The model under review builds one solid part; all positions refer to its coordinate system, in mm. A direction names the side the tool comes from. Coordinates: 2 decimals unless noted, no trailing zeros. Write each loop counter-clockwise with the first axis right and the second up, starting at its lowest first coordinate (ties: lowest second). Pieces come first, ordered by that corner, then holes. Notation, with made-up numbers: M -1,80.25 L 15,80.25 A22 cw 15,116.25 Z; hole C -12,73 d10. An arc over 180 degrees is marked long. Answer as CSV lines item,"result". Start each with the question number.
from build123d import *

# Parameters (mm, degrees)
BOX002_W          = 25
BOX002_H          = 10
BOX002_DEPTH      = 25.45
BOX010_W          = 25
BOX010_H          = 1
BOX010_DEPTH      = 25.45
BOX_W             = 25
BOX_H             = 20
BOX_DEPTH         = 12
CYLINDER_R        = 51.5
CYLINDER_DEPTH    = 16
CYLINDER001_R     = 53.5
CYLINDER001_DEPTH = 16


with BuildPart() as cube002:
    # Box002 → Box002 (new body)
    with BuildSketch(Plane(origin=(40, -5, 2.55), x_dir=(1, 0, 0), z_dir=(0, 0, 1))):
        with Locations((12.5, 5)):
            Rectangle(BOX002_W, BOX002_H)
    extrude(amount=BOX002_DEPTH)


with BuildPart() as cube010:
    # Box010 → Box010 (new body)
    with BuildSketch(Plane(origin=(45, -0.5, -3.45), x_dir=(1, 0, 0), z_dir=(0, 0, 1))):
        with Locations((12.5, 0.5)):
            Rectangle(BOX010_W, BOX010_H)
    extrude(amount=BOX010_DEPTH)


with BuildPart() as obj1:
    # Box → Box (new body)
    with BuildSketch(Plane(origin=(40, -10, 2), x_dir=(1, 0, 0), z_dir=(0, 0, 1))):
        with Locations((12.5, 10)):
            Rectangle(BOX_W, BOX_H)
    extrude(amount=BOX_DEPTH)

    # Fusion: union Cube002, Cube010
    add(cube002.part)
    add(cube010.part)


with BuildPart() as cylinder_chico:
    # Cylinder → Cylinder (new body)
    with BuildSketch(Plane.XY):
        Circle(CYLINDER_R)
    extrude(amount=CYLINDER_DEPTH)


with BuildPart() as cut015021:
    # Cylinder001 → Cylinder001 (new body)
    with BuildSketch(Plane.XY):
        Circle(CYLINDER001_R)
    extrude(amount=CYLINDER001_DEPTH)

    # Cut: cut Cylinder_chico
    add(cylinder_chico.part, mode=Mode.SUBTRACT)

    # Cut015021: cut obj1
    add(obj1.part, mode=Mode.SUBTRACT)


solid = cut015021.part
1) To check wall thickness, follow line 1 (Y direction, x = 0, z = 10.25); line 2 (X direction, y = -25.5, z = 9); line 3 (X direction, y = 0, z = 10.75). State the ranges of each line that lie inside material, in increasing order. Write a range as [from, to].
2) Clearance check with flat-ended pins moving along their axes: pin 1 Ø0.9 at (x, y) = (52, 3.5) entering from +Z; pin 2 Ø2 at (x, y) = (51.5, -8) entering from -Z; pin 3 Ø3 at (y, z) = (28.5, 5.5) entering from -X; pin 4 Ø2 at (y, z) = (-3.5, 11.5) entering from -X. State where each tip first meets the part, or that it passes through.
3) Mouldability with a two-part tool opening along X and no side actions: class faces 1 (the cylindrical face through (-53.45, 2.35, 7.89)), 2 (the cylindrical face through (-51.45, 2.26, 7.89)), 3 (the flat face through (52, -7, 14)) as +X half, -X half, draft (parallel to the pull), parting line (faces both ways), or undercut.
4) Take a section at A-A on x = 0. Give the boundary of the cut face in (y, z).
5) Tool access review of faces 4 (the flat face through (52, -5, 2)), 5 (the flat face through (-48, 20, 16)): name each direction out of +Z, -Z, +X, -X, +Y, -Y from which nothing blocks a thin tool from reaching the whole face with its end or side.
6) Take a section at B-B on y = -45.5. Give the boundary of the cut face in (x, z), and give its area (3 significant figures).
7) Take a section at C-C on z = 5.5. Give the boundary of the cut face in (x, y), and give its area (3 significant figures).
Results:
1,line 1,"y = [-53.5, -51.5], [51.5, 53.5]"
1,line 2,"x = [-47.03, -44.74], [44.74, 47.03]"
1,line 3,"x = [-53.5, -51.5]"
2,pin 1,"stops at z = 2"
2,pin 2,"stops at z = 0"
2,pin 3,"stops at x = -46.19"
2,pin 4,"stops at x = -53.44"
3,face 1,"parting line"
3,face 2,"undercut"
3,face 3,"draft"
4,outline,"M -53.5,0 L -51.5,0 L -51.5,16 L -53.5,16 Z; M 51.5,0 L 53.5,0 L 53.5,16 L 51.5,16 Z"
5,face 4,"+X"
5,face 5,"+Z, +X, -X, +Y, -Y"
6,outline,"M -28.14,0 L -24.12,0 L -24.12,16 L -28.14,16 Z; M 24.12,0 L 28.14,0 L 28.14,16 L 24.12,16 Z"
6,area,"129 mm²"
7,outline,"M 50.52,-10 A51.5 cw long 50.52,10 L 52.56,10 A53.5 ccw long 52.56,-10 Z"
7,area,"619 mm²"
